Could you check a few things on this model? Use its own coordinates, in mm. Face numbers are marked on the shaded views. A direction names the side the tool comes from. Give positions to 0.01 mm unless a question says otherwise; leave off trailing zeros. Loops run counter-clockwise (first coordinate to the right, second up) from the corner with the lowest first, then second, coordinate; pieces in that order, holes last. Notation, with made-up numbers: (-27, 44.5) -> (-21, 44.5) arc R14 ccw to (-21, 57.5) -> close; hole circle Ø11 at (-16, -29.75). An arc over 180 degrees is marked (long way). Write each question's results on one line, items separated by ' | '. Start each with the question number.
Q1. If we section it at C-C, the plane x = -17.5: List the corners of the cut face in (y, z) for me.
Q2. If we section it at D-D, the plane z = -6.25: List the corners of the cut face in (x, y) for me.
Q3. Which directions (+Z, -Z, +X, -X, +Y, -Y) give clear straight access to the entire face, cutting with the end or side of a thin tool? Please do the marked faces 1 and 2.
Q4. If we section it at A-A, the plane x = -3.5: List the corners of the cut face in (y, z) for me, plus the area to 4 significant figures.
Q5. Will these pins go through, and if not, where does the flat tip stop? P1, Ø2.5, axis at x = 21, y = -8.5, coming from the -Z side; P2, Ø4.5, axis at x = -17.5, z = -6.5, coming from the +Y side.
Q6. If I drill on line 1 along X through (y, z) = (-11.85, -6.5); line 2 along X through (y, z) = (5, 1); line 3 along X through (y, z) = (-6.5, 2), over which ranges is the centre line in solid material (lowest first)?
Q7. If we section it at B-B, the plane y = -4.5: List the corners of the cut face in (x, z) for me.
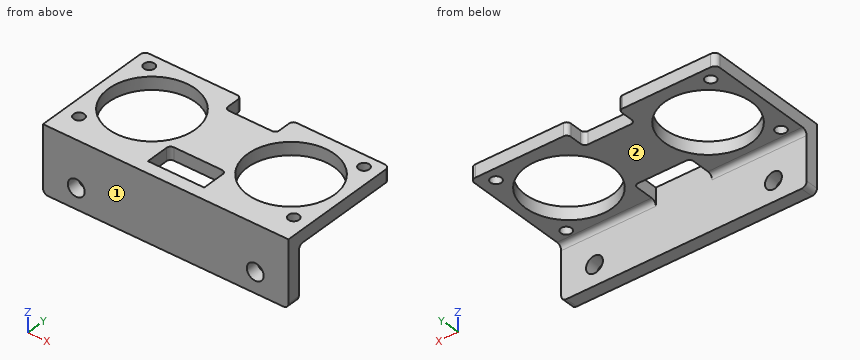
from build123d import *

# Parameters (mm, degrees)
SKETCH_1_R      = 1.05
SKETCH_1_R_2    = 8.5
EXTRUDE_1_DEPTH = 2.5
FILLET_1_R      = 0.8
SKETCH_2_W      = 48
SKETCH_2_H      = 13
SKETCH_2_R      = 1.65
EXTRUDE_2_DEPTH = 2.5
FILLET_2_R      = 1
FILLET_3_R      = 1


with BuildPart() as part:
    # 草图1 → 凸台-拉伸1 (new body)
    with BuildSketch(Plane.XY):
        Polygon((-24, 11), (-24, -11), (-5.5, -11), (-5.5, -5.7), (5.5, -5.7), (5.5, -11), (24, -11), (24, 11), (5, 11), (5, 7), (-5, 7), (-5, 11), align=None)
        with Locations((-21, -8.5)):
            Circle(SKETCH_1_R, mode=Mode.SUBTRACT)
        with Locations((21, -8.5)):
            Circle(SKETCH_1_R, mode=Mode.SUBTRACT)
        with Locations((-13.6, 0)):
            Circle(SKETCH_1_R_2, mode=Mode.SUBTRACT)
        with Locations((-21, 8.5)):
            Circle(SKETCH_1_R, mode=Mode.SUBTRACT)
        with Locations((13.6, 0)):
            Circle(SKETCH_1_R_2, mode=Mode.SUBTRACT)
        with Locations((21, 8.5)):
            Circle(SKETCH_1_R, mode=Mode.SUBTRACT)
    extrude(amount=EXTRUDE_1_DEPTH)

    # 圆角1
    fillet_1_edges = [part.edges().sort_by_distance(p)[0] for p in [
        (5, 11, 1.25),
        (5.5, -5.7, 1.25),
        (-5.5, -5.7, 1.25),
        (-5, 11, 1.25),
        (-5, 7, 1.25),
        (5, 7, 1.25),
    ]]
    fillet(fillet_1_edges, radius=FILLET_1_R)

    # 草图2 → 凸台-拉伸2 (add)
    with BuildSketch(Plane.XZ.offset(11)):
        with Locations((0, -4)):
            Rectangle(SKETCH_2_W, SKETCH_2_H)
        with Locations(Location((-17.5, -6.5, 0), (0, 0, 270))):
            Circle(SKETCH_2_R, mode=Mode.SUBTRACT)
        with Locations(Location((17.5, -6.5, 0), (0, 0, 270))):
            Circle(SKETCH_2_R, mode=Mode.SUBTRACT)
    extrude(amount=EXTRUDE_2_DEPTH)

    # 圆角2
    fillet_2_edges = [part.edges().sort_by_distance(p)[0] for p in [
        (14.75, -11, 0),
        (-14.75, -11, 0),
    ]]
    fillet(fillet_2_edges, radius=FILLET_2_R)

    # 圆角3
    fillet_3_edges = [part.edges().sort_by_distance(p)[0] for p in [
        (24, 11, 1.25),
        (-24, 11, 1.25),
        (-24, -12.25, -10.5),
        (24, -12.25, -10.5),
    ]]
    fillet(fillet_3_edges, radius=FILLET_3_R)


solid = part.part
Final values:
1) outline: (-13.5, -10.5) -> (-11, -10.5) -> (-11, -8.15) -> (-13.5, -8.15) -> close; (-13.5, -4.85) -> (-11, -4.85) -> (-11, -1) arc R1 cw to (-10, 0) -> (-7.55, 0) -> (-7.55, 2.5) -> (-13.5, 2.5) -> close; (7.55, 0) -> (11, 0) -> (11, 2.5) -> (7.55, 2.5) -> close
2) outline: (-24, -13.5) -> (-19.13, -13.5) -> (-19.13, -11) -> (-24, -11) -> close; (-15.87, -13.5) -> (15.87, -13.5) -> (15.87, -11) -> (-15.87, -11) -> close; (19.13, -13.5) -> (24, -13.5) -> (24, -11) -> (19.13, -11) -> close
3) face 1: +Z, -Z, +X, -X, -Y | face 2: -Z, +X, -X, +Y
4) outline: (-13.5, -10.5) -> (-11, -10.5) -> (-11, 2.5) -> (-13.5, 2.5) -> close; (-5.7, 0) -> (7, 0) -> (7, 2.5) -> (-5.7, 2.5) -> close | area: 64.25 mm²
5) P1: stops at z = 0 | P2: stops at y = -11
6) line 1: x = -24 to -19.15, -15.85 to 15.85, 19.15 to 24 | line 2: x = -24 to -20.47, -6.73 to 6.73, 20.47 to 24 | line 3: x = -24 to -19.08, -8.12 to -5.5, 5.5 to 8.12, 19.08 to 24
7) outline: (-24, 0) -> (-20.81, 0) -> (-20.81, 2.5) -> (-24, 2.5) -> close; (-6.39, 0) -> (6.39, 0) -> (6.39, 2.5) -> (-6.39, 2.5) -> close; (20.81, 0) -> (24, 0) -> (24, 2.5) -> (20.81, 2.5) -> close
